Read the model definition and answer for the solid it produces. Units are mm, in the model's axes. Face numbers are marked on the shaded views. A direction names the side the tool comes from. Give positions to 0.01 mm unless a question says otherwise; leave off trailing zeros. Order: outer loops, then holes, each group sorted by start corner. A loop starts at its lowest first (then second) coordinate and runs counter-clockwise, first axis right, second up. Notation, with made-up numbers: M 47,25.5 L 106,25.5 A14 cw 106,43.5 Z; hole C 1,-34.5 d3. An arc over 180 degrees is marked long. One line per item, written item: value. Start each with the question number.
from build123d import *

# Parameters (mm, degrees)
PAD015_DEPTH      = 0.5
BOX039_W          = 18
BOX039_H          = 10
BOX039_DEPTH      = 11
BOX038_W          = 14
BOX038_H          = 10
BOX038_DEPTH      = 10
CYLINDER036_R     = 1.25
CYLINDER036_DEPTH = 8
CYLINDER037_R     = 1.25
CYLINDER037_DEPTH = 8
CYLINDER014_R     = 1.9
CYLINDER014_DEPTH = 20
CYLINDER015_R     = 1.9
CYLINDER015_DEPTH = 20
BOX015_W          = 13
BOX015_H          = 4.9
BOX015_DEPTH      = 2.5
BOX035_W          = 13
BOX035_H          = 24.1
BOX035_DEPTH      = 20
BOX014_W          = 13
BOX014_H          = 4.9
BOX014_DEPTH      = 2.5
BOX016_W          = 18
BOX016_H          = 35.9
BOX016_DEPTH      = 20
FILLET008_R       = 1.3
FILLET010_R       = 1.5
POCKET020_DEPTH   = 0.5
POCKET021_DEPTH   = 0.5


with BuildPart() as pad015:
    # Sketch046 → Pad015 (new body)
    with BuildSketch(Plane(origin=(53.5, 6, 2.5), x_dir=(0, 1, 0), z_dir=(1, 0, 0))):
        Polygon((4.75, 6.75), (-4.75, 6.75), (-4.75, 13.5), (-7, 13.5), (-7, 14.25), (-4.75, 14.25), (-4.75, 15.75), (-3, 15.75), (-3, 17), (-1.85, 17), (-1.85, 15.75), (3.25, 15.75), (4.75, 14.25), (7, 14.25), (7, 13.5), (4.75, 13.5), align=None)
    extrude(amount=PAD015_DEPTH)


with BuildPart() as obj1:
    # Box039 → Box039 (new body)
    with BuildSketch(Plane(origin=(49, 20, 3), x_dir=(1, 0, 0), z_dir=(0, 0, 1))):
        with Locations((9, 5)):
            Rectangle(BOX039_W, BOX039_H)
    extrude(amount=BOX039_DEPTH)


with BuildPart() as obj2:
    # Box038 → Box038 (new body)
    with BuildSketch(Plane(origin=(57, -14, -4), x_dir=(1, 0, 0), z_dir=(0, 0, 1))):
        with Locations((7, 5)):
            Rectangle(BOX038_W, BOX038_H)
    extrude(amount=BOX038_DEPTH)


with BuildPart() as cylinder036:
    # Cylinder036 → Cylinder036 (new body)
    with BuildSketch(Plane(origin=(57, -106, 14), x_dir=(1, 0, 0), z_dir=(0, 0, 1))):
        Circle(CYLINDER036_R)
    extrude(amount=CYLINDER036_DEPTH)


with BuildPart() as fusion036:
    # Cylinder037 → Cylinder037 (new body)
    with BuildSketch(Plane(origin=(57, -134, 14), x_dir=(1, 0, 0), z_dir=(0, 0, 1))):
        Circle(CYLINDER037_R)
    extrude(amount=CYLINDER037_DEPTH)

    # Fusion036: union Cylinder036
    add(cylinder036.part)


with BuildPart() as cylinder014:
    # Cylinder014 → Cylinder014 (new body)
    with BuildSketch(Plane(origin=(48, -132.8, 1), x_dir=(1, 0, 0), z_dir=(0, 0, 1))):
        Circle(CYLINDER014_R)
    extrude(amount=CYLINDER014_DEPTH)


with BuildPart() as fusion035:
    # Cylinder015 → Cylinder015 (new body)
    with BuildSketch(Plane(origin=(48, -107.2, 1), x_dir=(1, 0, 0), z_dir=(0, 0, 1))):
        Circle(CYLINDER015_R)
    extrude(amount=CYLINDER015_DEPTH)

    # Fusion035: union Cylinder014
    add(cylinder014.part)


with BuildPart() as box015:
    # Box015 → Box015 (new body)
    with BuildSketch(Plane(origin=(50, -108.5, 16), x_dir=(1, 0, 0), z_dir=(0, 0, 1))):
        with Locations((6.5, 2.45)):
            Rectangle(BOX015_W, BOX015_H)
    extrude(amount=BOX015_DEPTH)


with BuildPart() as obj3:
    # Box035 → Box035 (new body)
    with BuildSketch(Plane(origin=(50, -132.1, 1), x_dir=(1, 0, 0), z_dir=(0, 0, 1))):
        with Locations((6.5, 12.05)):
            Rectangle(BOX035_W, BOX035_H)
    extrude(amount=BOX035_DEPTH)


with BuildPart() as fusion034:
    # Box014 → Box014 (new body)
    with BuildSketch(Plane(origin=(50, -136.5, 16), x_dir=(1, 0, 0), z_dir=(0, 0, 1))):
        with Locations((6.5, 2.45)):
            Rectangle(BOX014_W, BOX014_H)
    extrude(amount=BOX014_DEPTH)

    # Fusion034: union Box015, obj3
    add(box015.part)
    add(obj3.part)


with BuildPart() as obj4:
    # Box016 → Box016 (new body)
    with BuildSketch(Plane(origin=(45, -138, 1), x_dir=(1, 0, 0), z_dir=(0, 0, 1))):
        with Locations((9, 17.95)):
            Rectangle(BOX016_W, BOX016_H)
    extrude(amount=BOX016_DEPTH)

    # Cut012: cut Fusion034
    add(fusion034.part, mode=Mode.SUBTRACT)

    # Cut013: cut Fusion035
    add(fusion035.part, mode=Mode.SUBTRACT)

    # Cut016: cut Fusion036
    add(fusion036.part, mode=Mode.SUBTRACT)

    # Fillet008
    fillet008_edges = [obj4.edges().sort_by_distance(p)[0] for p in [
        (45, -138, 11),
        (45, -120.05, 21),
        (45, -102.1, 11),
        (63, -138, 11),
        (54, -138, 21),
        (54, -102.1, 21),
        (63, -105.05, 21),
        (63, -135.05, 21),
        (63, -102.1, 11),
    ]]
    fillet(fillet008_edges, radius=FILLET008_R)


with BuildPart() as obj4_1:
    # Fillet008 placement: moved
    add(obj4.part.moved(Location((5, 126, 2))))

    # Cut017: cut obj2
    add(obj2.part, mode=Mode.SUBTRACT)


with BuildPart() as obj4_2:
    # Cut017 placement: moved
    add(obj4_1.part.moved(Location((-1, 0, 0))))

    # Cut019: cut obj1
    add(obj1.part, mode=Mode.SUBTRACT)

    # Fillet010
    fillet010_edges = [obj4_2.edges().sort_by_distance(p)[0] for p in [
        (49, 21.3, 14),
        (49, 20, 8.5),
        (49.380761, 23.519239, 14),
        (58, 23.9, 14),
        (66.619239, 23.519239, 14),
        (67, 21.3, 14),
        (56, -12, 4.5),
        (60.85, -12, 6),
        (67, 20, 8.5),
        (67, -8.4, 6),
        (66.619239, -11.619239, 6),
    ]]
    fillet(fillet010_edges, radius=FILLET010_R)


with BuildPart() as obj4_3:
    # Fillet010 placement: moved
    add(obj4_2.part.moved(Location((0, 0, -1))))

    # Sketch044 → Pocket020 (cut)
    with BuildSketch(Plane(origin=(0, -12, -1), x_dir=(1, 0, 0), z_dir=(0, -1, 0))):
        Polygon((54.3, 19.95), (54.3, 17.95), (60.3, 17.95), (60.3, 16.95), (62.3, 18.95), (60.3, 20.95), (60.3, 19.95), align=None)
    extrude(amount=-POCKET020_DEPTH, mode=Mode.SUBTRACT)

    # Sketch045 → Pocket021 (cut)
    with BuildSketch(Plane(origin=(0, 23.9, -1), x_dir=(-1, 0, 0), z_dir=(0, 1, 0))):
        Polygon((-60.3, 19.95), (-54.3, 19.95), (-54.3, 17.95), (-60.3, 17.95), (-60.3, 16.95), (-62.3, 18.95), (-60.3, 20.95), align=None)
    extrude(amount=-POCKET021_DEPTH, mode=Mode.SUBTRACT)

    # Cut056: cut Pad015
    add(pad015.part, mode=Mode.SUBTRACT)


solid = obj4_3.part
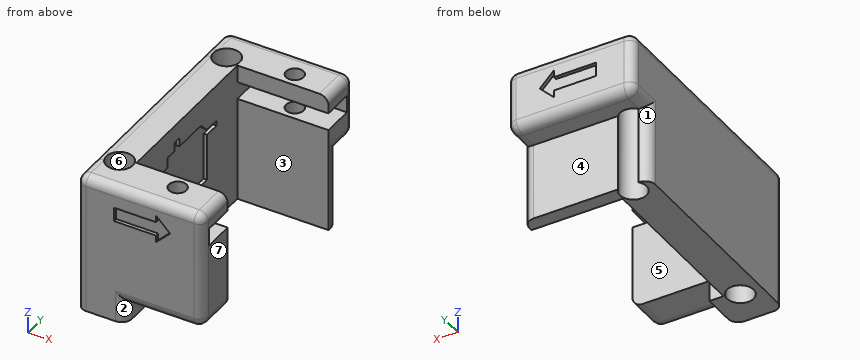
Q1. Determine the mould class of the marked faces 5, 6 and 7 for opening direction X: released by +X, released by -X, zero draft, split by the parting line, or undercut.
Q2. Consider probe 1 along X at (y, z) = (-8, 15.85); probe 2 along Y at (x, z) = (61, 15.6); probe 3 along Y at (x, z) = (64.75, 18.75). Determine where each line is inside the solid, lowest interval first.
Q3. A tool of negligible diameter and unlimited length cuts with its end or side. For the marked faces 1, 2, 3 and 4, from which of +Z, -Z, +X, -X, +Y, -Y can it reach the whole face along a straight path? Write none if from no direction.
Q4. Find section A-A, the plane x = 52. Give the vertices of the cut face in (y, z).
Q5. Each of these flat-tipped pins is pushed along its axis until it touches: pin 1 (1.9 mm diameter, centred on x = 56, y = 21, fed in from -Z); pin 2 (4.5 mm diameter, centred on x = 57, z = 17.5, fed in from -Y); pin 3 (3 mm diameter, centred on x = 56.5, z = 12.5, fed in from +Y). Where does it stop, or does it pass through?
Q6. Find section B-B, the plane z = 17.5. Give the vertices of the cut face in (x, y).
Evaluation:
1. face 5: zero draft
1. face 6: undercut
1. face 7: released by +X
2. probe 1: 49 to 50.53, 53.47 to 59.75, 62.25 to 67
2. probe 2: -12 to -9.25, -6.75 to -6.1, 18 to 18.75, 21.25 to 23.9
2. probe 3: -12 to -10.5, 22.4 to 23.9
3. face 1: -Z, -X, +Y
3. face 2: -Z, +X, -Y
3. face 3: +Z, -Z, +X
3. face 4: -Z, +X, -X, +Y
4. outline: M -12,2 L -8.7,2 L -8.7,22 L -10.7,22 A1.3 ccw -12,20.7 Z; M -4.9,2 L 16.9,2 L 16.9,22 L -4.9,22 Z; M 20.7,13 L 22.4,13 A1.5 ccw 23.9,14.5 L 23.9,20.7 A1.3 ccw 22.6,22 L 20.7,22 Z
5. pin 1: z = 13
5. pin 2: y = -12
5. pin 3: y = 23.81
6. outline: M 49,-10.7 A1.3 ccw 50.3,-12 L 54.3,-12 L 54.3,-11.5 L 61.85,-11.5 L 61.85,-12 L 65.7,-12 A1.3 ccw 67,-10.7 L 67,-10.5 L 54,-10.5 L 54,1.25 L 53.5,1.25 L 53.5,10 L 54,10 L 54,22.4 L 67,22.4 L 67,22.6 A1.3 ccw 65.7,23.9 L 61.85,23.9 L 61.85,23.4 L 54.3,23.4 L 54.3,23.9 L 50.3,23.9 A1.3 ccw 49,22.6 Z; hole C 52,-6.8 d3.8; hole C 52,18.8 d3.8
